For this review, use the dimensioned drawing (mm, ordinates from the lowest corner) and the shaded views. A direction names the side the tool comes from. Round coordinates to 2 decimals unless told otherwise and drop trailing zeros. Loops run counter-clockwise (first coordinate to the right, second up) from the corner with the lowest first, then second, coordinate; pieces in that order, holes last. Notation, with made-up numbers: (70, -19) -> (79, -19) arc R22 ccw to (79, -9) -> close; hole circle Ø5 at (-21, -8). An arc over 180 degrees is marked (long way). Write each question's results on one line, items separated by ' | '. Start each with the question number.
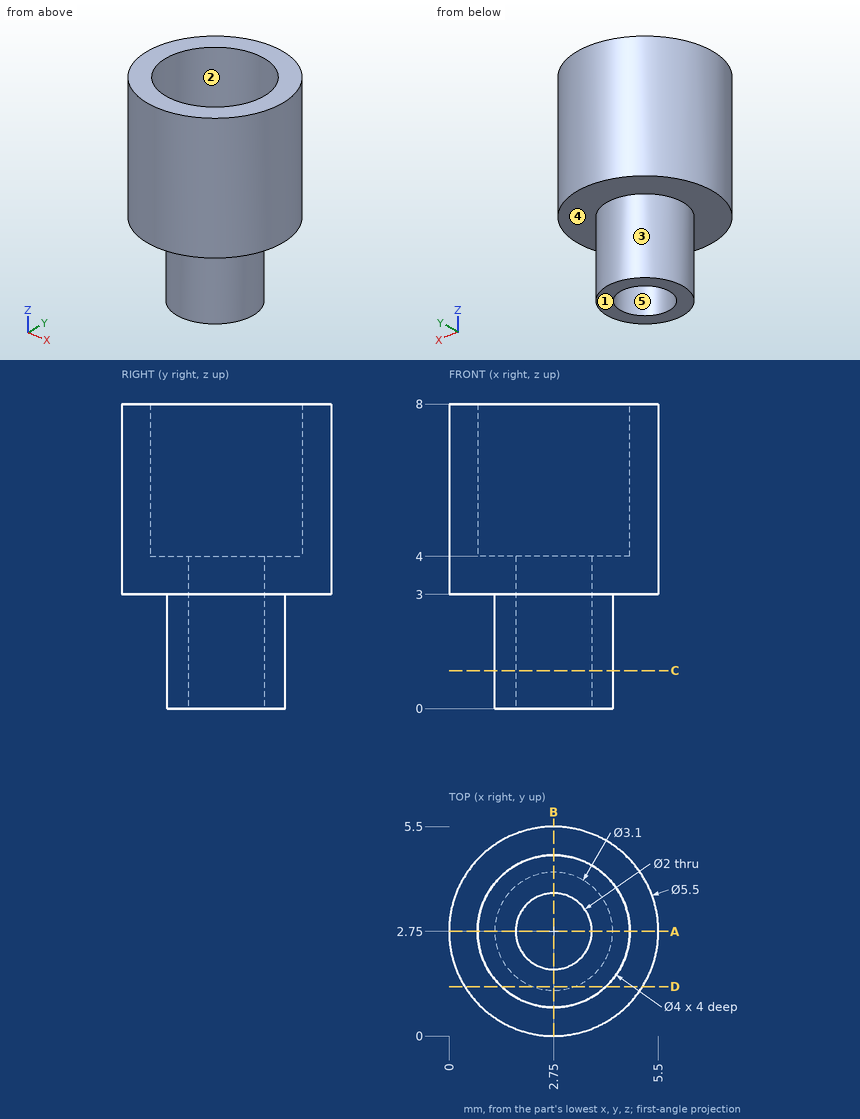
1) Take a section at D-D (y = 1.3). Write out the cut boundary in (x, z), plus the area to 3 significant figures.
2) For the marked faces 4 and 5, list the 3-axis set-ups (+Z, -Z, +X, -X, +Y, -Y) from which the entire face can be reached by the end or side of a thin tool; tool diameter is ignored.
3) The part is to be moulded in two halves that separate along Y. For the marked faces 1, 2 and 3, say which applies: +Y half, -Y half, draft (parallel to the pull), parting line (faces both ways), or undercut.
4) To check wall thickness, follow line 1 (X direction, y = 2.7, z = 1.5); line 2 (X direction, y = 2.85, z = 5.5). State the ranges of each line that lie inside material, in increasing order. Write a range as from..to.
5) Insertion check: pin 1 (3 mm diameter, centred on y = 1, z = 5, fed in from -X); pin 2 (1 mm diameter, centred on x = 1, z = 4, fed in from -Y); pin 3 (3 mm diameter, centred on x = 2.75, y = 2.75, fed in from +Z). Each pin has a flat end and moves straight along its axis. Give the tip position at first contact, or say it passes through.
6) Take a section at A-A (y = 2.75). Write out the cut boundary in (x, z), plus the area to 3 significant figures.
7) Take a section at C-C (z = 1). Write out the cut boundary in (x, y), plus the area to 3 significant figures.
Geometry check:
1) outline: (0.41, 3) -> (2.2, 3) -> (2.2, 0) -> (3.3, 0) -> (3.3, 3) -> (5.09, 3) -> (5.09, 8) -> (4.13, 8) -> (4.13, 4) -> (1.37, 4) -> (1.37, 8) -> (0.41, 8) -> close | area: 15.6 mm^2
2) face 4: -Z | face 5: +Z, -Z
3) face 1: draft | face 2: undercut | face 3: parting line
4) line 1: x = 1.2..1.75, 3.75..4.3 | line 2: x = 0..0.75, 4.75..5.5
5) pin 1: stops at x = 0.01 | pin 2: stops at y = 0.3 | pin 3: stops at z = 4
6) outline: (0, 3) -> (1.2, 3) -> (1.2, 0) -> (1.75, 0) -> (1.75, 4) -> (0.75, 4) -> (0.75, 8) -> (0, 8) -> close; (3.75, 0) -> (4.3, 0) -> (4.3, 3) -> (5.5, 3) -> (5.5, 8) -> (4.75, 8) -> (4.75, 4) -> (3.75, 4) -> close | area: 12.8 mm^2
7) outline: circle Ø3.1 at (2.75, 2.75); hole circle Ø2 at (2.75, 2.75) | area: 4.41 mm^2
